```python
from build123d import *

# Parameters (mm, degrees)
CHAMFER1_SIZE        = 0.2
CHAMFER2_SIZE        = 0.2
CHAMFER3_SIZE        = 0.5
CHAMFER4_SIZE        = 0.5
FILLET1_R            = 0.2
FILLET2_R            = 0.2
SKETCH11_W           = 8
SKETCH11_H           = 3
BOSS_EXTRUDE10_DEPTH = 1.8
FILLET19_RADIUS      = 1.5
FILLET19_LENGTH      = 1.8
FILLET20_RADIUS      = 1.5
FILLET20_LENGTH      = 1.8
FILLET21_R           = 0.1
SKETCH21_W           = 0.9
SKETCH21_H           = 1.5


with BuildPart() as part:
    # Sketch1 → Revolve1 (revolve)
    with BuildSketch(Plane.XY, mode=Mode.PRIVATE) as revolve1_sk:
        Polygon((0, 0), (81, 0), (81, 4), (66, 4), (66, 5), (15, 5), (15, 4), (0, 4), align=None)
    revolve(revolve1_sk.sketch.rotate(Axis((0, 0, 0), (1, 0, 0)), 90), axis=Axis((0, 0, 0), (1, 0, 0)))

    # Chamfer1
    chamfer1_edges = [part.edges().sort_by_distance(p)[0] for p in [
        (66, 0, -5),
    ]]
    chamfer(chamfer1_edges, length=CHAMFER1_SIZE)

    # Chamfer2
    chamfer2_edges = [part.edges().sort_by_distance(p)[0] for p in [
        (15, 0, -5),
    ]]
    chamfer(chamfer2_edges, length=CHAMFER2_SIZE)

    # Chamfer3
    chamfer3_edges = [part.edges().sort_by_distance(p)[0] for p in [
        (0, 0, -4),
    ]]
    chamfer(chamfer3_edges, length=CHAMFER3_SIZE)

    # Chamfer4
    chamfer4_edges = [part.edges().sort_by_distance(p)[0] for p in [
        (81, 0, -4),
    ]]
    chamfer(chamfer4_edges, length=CHAMFER4_SIZE)

    # Fillet1
    fillet1_edges = [part.edges().sort_by_distance(p)[0] for p in [
        (15, 0, -4),
    ]]
    fillet(fillet1_edges, radius=FILLET1_R)

    # Fillet2
    fillet2_edges = [part.edges().sort_by_distance(p)[0] for p in [
        (66, 0, -4),
    ]]
    fillet(fillet2_edges, radius=FILLET2_R)


with BuildPart() as body_2:
    # Sketch11 → Boss-Extrude10 (new body)
    with BuildSketch(Plane.XY.offset(4)):
        with Locations((9, 0)):
            Rectangle(SKETCH11_W, SKETCH11_H)
    extrude(amount=-BOSS_EXTRUDE10_DEPTH)

    # Fillet19: full round fillet: the end face becomes a half cylinder, R = half its width
    fillet19_face = Plane((5, 0, 3.1), x_dir=(0, 0, 1), z_dir=(-1, 0, 0))  # on the end face: x along it, z out of the body
    fillet19_slab = fillet19_face.offset(-FILLET19_RADIUS / 2) * Box(FILLET19_LENGTH, 2 * FILLET19_RADIUS, FILLET19_RADIUS, mode=Mode.PRIVATE)  # the body's end, R deep
    fillet19_round = Plane((6.5, 0, 3.1), x_dir=(-1, 0, 0), z_dir=(0, 0, 1)) * Cylinder(FILLET19_RADIUS, FILLET19_LENGTH, mode=Mode.PRIVATE)  # its axis R under the face
    add(fillet19_slab - fillet19_round, mode=Mode.SUBTRACT)

    # Fillet20: full round fillet: the end face becomes a half cylinder, R = half its width
    fillet20_face = Plane((13, 0, 3.1), x_dir=(0, 0, -1), z_dir=(1, 0, 0))  # on the end face: x along it, z out of the body
    fillet20_slab = fillet20_face.offset(-FILLET20_RADIUS / 2) * Box(FILLET20_LENGTH, 2 * FILLET20_RADIUS, FILLET20_RADIUS, mode=Mode.PRIVATE)  # the body's end, R deep
    fillet20_round = Plane((11.5, 0, 3.1), x_dir=(1, 0, 0), z_dir=(0, 0, -1)) * Cylinder(FILLET20_RADIUS, FILLET20_LENGTH, mode=Mode.PRIVATE)  # its axis R under the face
    add(fillet20_slab - fillet20_round, mode=Mode.SUBTRACT)

    # Fillet21
    fillet21_edges = [body_2.edges().sort_by_distance(p)[0] for p in [
        (9, -1.5, 2.2),
        (5, 0, 2.2),
        (9, 1.5, 2.2),
        (13, 0, 2.2),
    ]]
    fillet(fillet21_edges, radius=FILLET21_R)


with BuildPart() as part_1:
    add(part.part)

    # Combine6: cut body 2
    add(body_2.part, mode=Mode.SUBTRACT)

    # Sketch21 → Cut-Revolve3 (revolve, cut)
    with BuildSketch(Plane.XY, mode=Mode.PRIVATE) as cut_revolve3_sk:
        with Locations((15.55, 4.25)):
            Rectangle(SKETCH21_W, SKETCH21_H)
    revolve(cut_revolve3_sk.sketch.rotate(Axis((0, 0, 0), (1, 0, 0)), 270), axis=Axis((0, 0, 0), (1, 0, 0)), mode=Mode.SUBTRACT)


solid = part_1.part
```
CAD build for the part. Positions are in the model's coordinates, mm. A direction names the side the tool comes from. Round coordinates to 2 decimals unless told otherwise and drop trailing zeros. Order: outer loops, then holes, each group sorted by start corner. A loop starts at its lowest first (then second) coordinate and runs counter-clockwise, first axis right, second up.
Q1. Slice it at B-B (x = 76.5). Write the cut outline in (y, z), and give its area (3 significant figures).
Q2. Drop flat-ended pins along their axis: pin 1 (4 mm diameter, centred on x = 14.5, z = 2, fed in from +Y); pin 2 (1.1 mm diameter, centred on x = 8.5, z = 2.5, fed in from +Y); pin 3 (3 mm diameter, centred on x = 10, y = -0.5, fed in from +Z). Give the stop position or say it passes through.
Q3. Two-plate mould, pull along Y, no slides. Class faces 1 (the flat face through (66, 4, -2)), 2 (the cylindrical face through (41, 0, -5)), 3 (the flat face through (9, 1.5, 3)): pulls with the +Y half, pulls with the -Y half, needs draft (parallel to the pull), parting line crosses it, or undercut.
Q4. Which spindle directions (+Z, -Z, +X, -X, +Y, -Y) get a long thin tool onto all of the face, cutting with end or side? Do faces 4 (the cylindrical face through (73.25, 3.905, -0.867)), 5 (the flat face through (9, -1.5, 3)), 6 (the cylindrical face through (15.556, -3.417, 0.759)), 7 (the cylindrical face through (7.5, 2.4, -3.2)), 8 (the flat face through (81, 0, 0)). Say none if no direction does.
Q5. Wall check: L1, parallel to Y at x = 19, z = -3; L2, parallel to X at y = -3.75, z = 1. Give the ranges that are in metal, low to high.
Results below:
1. outline: circle Ø8 at (0, 0)
1. area: 50.3 mm2
2. pin 1: stops at y = 4.95
2. pin 2: stops at y = 3.49
2. pin 3: stops at z = 3.71
3. face 1: needs draft
3. face 2: parting line crosses it
3. face 3: undercut
4. face 4: +X
4. face 5: +Z
4. face 6: none
4. face 7: -X
4. face 8: +Z, -Z, +X, +Y, -Y
5. L1: y = -4 to 4
5. L2: x = 0.38 to 15.1, 16 to 80.62
